```python
from build123d import *

# Parameters (mm, degrees)
SKETCH068_R     = 1.25
PAD036_DEPTH    = 4
PAD037_DEPTH    = 8
POCKET027_DEPTH = 8
PAD038_DEPTH    = 4
PAD039_DEPTH    = 4
PAD040_DEPTH    = 4
PAD041_DEPTH    = 4
SKETCH076_R     = 1.75
POCKET028_DEPTH = 4
FILLET006_R     = 1
CHAMFER_SIZE    = 1


with BuildPart() as part:
    # Sketch068 → Pad036 (new body)
    with BuildSketch(Plane.XY):
        Polygon((0, 0), (-44, 0), (-44, -5), (-32, -5), (-32, -28), (-44, -28), (-44, -33), (0, -33), (0, -28), (-12, -28), (-12, -5), (0, -5), align=None)
        with Locations((-6, -1.8)):
            Circle(SKETCH068_R, mode=Mode.SUBTRACT)
        with Locations((-38, -31.2)):
            Circle(SKETCH068_R, mode=Mode.SUBTRACT)
        with Locations((-6, -31.2)):
            Circle(SKETCH068_R, mode=Mode.SUBTRACT)
        with Locations((-38, -1.8)):
            Circle(SKETCH068_R, mode=Mode.SUBTRACT)
    extrude(amount=PAD036_DEPTH)

    # Sketch069 → Pad037 (join)
    with BuildSketch(Plane.XY.offset(4)):
        Polygon((0, 0), (-44, 0), (-44, -5), (-31, -5), (-31, -28), (-44, -28), (-44, -33), (0, -33), (0, -28), (-13, -28), (-13, -5), (0, -5), align=None)
    extrude(amount=PAD037_DEPTH)

    # Sketch070 → Pocket027 (cut)
    with BuildSketch(Plane.XY.offset(3)):
        Polygon((-42.5, -1.5), (-42.5, -3.5), (-29, -3.5), (-29, -5), (-29, -29.5), (-42.5, -29.5), (-42.5, -31.5), (-1.5, -31.5), (-1.5, -29.5), (-15, -29.5), (-15, -3.5), (-1.5, -3.5), (-1.5, -1.5), align=None)
    extrude(amount=POCKET027_DEPTH, mode=Mode.SUBTRACT)

    # Sketch072 → Pad038 (join)
    with BuildSketch(Plane(origin=(-38, 0, 12), x_dir=(1, 0, 0), z_dir=(0, 0, 1))):
        Polygon((-1.8, 0), (-1.8, 2), (-0.7, 2), (-0.7, 3.5), (-3.8, 3.5), (-3.8, 0), align=None)
        Polygon((0.7, 2), (1.8, 2), (1.8, 0), (3.8, 0), (3.8, 3.5), (0.7, 3.5), align=None)
    extrude(amount=-PAD038_DEPTH)

    # Sketch073 → Pad039 (join)
    with BuildSketch(Plane(origin=(-38, 0, 0), x_dir=(1, 0, 0), z_dir=(0, 0, 1))):
        Polygon((-1.8, 0), (-1.8, 2), (-0.7, 2), (-0.7, 3.5), (-3.8, 3.5), (-3.8, 0), align=None)
        Polygon((0.7, 2), (1.8, 2), (1.8, 0), (3.8, 0), (3.8, 3.5), (0.7, 3.5), align=None)
    extrude(amount=PAD039_DEPTH)

    # Sketch074 → Pad040 (join)
    with BuildSketch(Plane(origin=(-6, 0, 0), x_dir=(1, 0, 0), z_dir=(0, 0, 1))):
        Polygon((-1.8, 0), (-1.8, 2), (-0.7, 2), (-0.7, 3.5), (-3.8, 3.5), (-3.8, 0), align=None)
        Polygon((0.7, 2), (1.8, 2), (1.8, 0), (3.8, 0), (3.8, 3.5), (0.7, 3.5), align=None)
    extrude(amount=PAD040_DEPTH)

    # Sketch075 → Pad041 (join)
    with BuildSketch(Plane(origin=(-6, 0, 12), x_dir=(1, 0, 0), z_dir=(0, 0, 1))):
        Polygon((-1.8, 0), (-1.8, 2), (-0.7, 2), (-0.7, 3.5), (-3.8, 3.5), (-3.8, 0), align=None)
        Polygon((0.7, 2), (1.8, 2), (1.8, 0), (3.8, 0), (3.8, 3.5), (0.7, 3.5), align=None)
    extrude(amount=-PAD041_DEPTH)

    # Sketch076 → Pocket028 (cut)
    with BuildSketch(Plane.YZ):
        with Locations((-30.5, 9.5)):
            Circle(SKETCH076_R)
        with Locations((-30.5, 2.5)):
            Circle(SKETCH076_R)
        with Locations((-2.5, 2.5)):
            Circle(SKETCH076_R)
        with Locations((-2.5, 9.5)):
            Circle(SKETCH076_R)
    extrude(amount=-POCKET028_DEPTH, mode=Mode.SUBTRACT)

    # Fillet006
    fillet006_edges = [part.edges().sort_by_distance(p)[0] for p in [
        (-9.8, 3.5, 2),
        (-2.2, 3.5, 2),
        (-2.2, 3.5, 10),
        (-9.8, 3.5, 10),
        (-34.2, 3.5, 10),
        (-41.8, 3.5, 10),
        (-41.8, 3.5, 2),
        (-34.2, 3.5, 2),
    ]]
    fillet(fillet006_edges, radius=FILLET006_R)

    # Chamfer
    chamfer_edges = [part.edges().sort_by_distance(p)[0] for p in [
        (-5.3, 3.5, 2),
        (-6.7, 3.5, 2),
        (-5.3, 3.5, 10),
        (-6.7, 3.5, 10),
        (-37.3, 3.5, 2),
        (-38.7, 3.5, 2),
        (-38.7, 3.5, 10),
        (-37.3, 3.5, 10),
    ]]
    chamfer(chamfer_edges, length=CHAMFER_SIZE)


with BuildPart() as part_1:
    # Body011 placement: moved
    add(part.part.moved(Location((5, 11, 16.4))))


solid = part_1.part
```
Geometry check sheet. Reference: the model listing, model coordinates, mm. A direction names the side the tool comes from. Round coordinates to 2 decimals unless told otherwise and drop trailing zeros. Order: outer loops, then holes, each group sorted by start corner. A loop starts at its lowest first (then second) coordinate and runs counter-clockwise, first axis right, second up. Notation, with made-up numbers: (-33, 32.25) -> (-3, 32.25) arc R33 cw to (-3, 63.25) -> close; hole circle Ø1 at (36.5, -3). An arc over 180 degrees is marked (long way). Return JSON: item names as keys, results as strings. Group by question number.
Q1. Section check A-A, the plane x = -33. Record the boundary of the cut face in (y, z).
Q2. Release check for a two-part mould opening along X. For faces 5 (the flat face through (-39, -19, 22)), 6 (the flat face through (-30, 13, 24.4)), 7 (the flat face through (-34, 13, 26)) record: released by +X, released by -X, zero draft, split by the parting line, or undercut.
Q3. Gauge pin test, flat ends, axial feed: pin 1 (1.5 mm diameter, centred on x = -26, z = 22.5, fed in from +Y); pin 2 (1.5 mm diameter, centred on y = -1.5, z = 24, fed in from -X); pin 3 (1.5 mm diameter, centred on y = 0.5, z = 21, fed in from +X); pin 4 (2 mm diameter, centred on y = 11.5, z = 26, fed in from +X). Record the tip position at first contact, or that the pin passes through.
Q4. Tool access check on faces 1 (the flat face through (-19, -5, 19.4)), 2 (the cylindrical face through (-0.328, 10.254, 18.372)), 3 (the flat face through (0.2, 14, 18.4)), 4 (the flat face through (-26.5, -5.3, 20.4)). Record the directions out of +Z, -Z, +X, -X, +Y, -Y that give a thin tool (end or side, any length) a straight path to the whole face; none if there is none.
Q5. Section check B-B, the plane y = -2.5. Record the boundary of the cut face in (x, z).
Q6. Section check C-C, the plane x = -17. Record the boundary of the cut face in (y, z).
Q7. Material ranges on probe 1 along Y at (x, z) = (-1, 17.3); probe 2 along X at (y, z) = (9.2, 19); probe 3 along Y at (x, z) = (-1, 19.5), recorded low to high. Write a range as from..to.
Q8. Section check D-D, the plane z = 22.25. Record the boundary of the cut face in (x, y), plus the area to 3 significant figures.
Numbers:
{
 "1": {"outline": "(-22, 16.4) -> (-21.45, 16.4) -> (-21.45, 20.4) -> (-20.5, 20.4) -> (-20.5, 27.4) -> (-18.5, 27.4) -> (-18.5, 19.4) -> (-18.95, 19.4) -> (-18.95, 16.4) -> (-17, 16.4) -> (-17, 28.4) -> (-22, 28.4) -> close; (6, 16.4) -> (7.95, 16.4) -> (7.95, 19.4) -> (7.5, 19.4) -> (7.5, 27.4) -> (9.5, 27.4) -> (9.5, 20.4) -> (10.45, 20.4) -> (10.45, 16.4) -> (11, 16.4) -> (11, 28.4) -> (6, 28.4) -> close"},
 "2": {"face 5": "released by -X", "face 6": "zero draft", "face 7": "undercut"},
 "3": {"pin 1": "y = 11", "pin 2": "x = -26", "pin 3": "x = -7", "pin 4": "x = 5"},
 "4": {"face 1": "none", "face 2": "-Z", "face 3": "+Z, -Z, +Y", "face 4": "+Z, -X"},
 "5": {"outline": "(-27, 16.4) -> (-7, 16.4) -> (-7, 20.4) -> (-8, 20.4) -> (-8, 28.4) -> (-26, 28.4) -> (-26, 20.4) -> (-27, 20.4) -> close; hole (-24, 19.4) -> (-10, 19.4) -> (-10, 27.4) -> (-24, 27.4) -> close"},
 "6": {"outline": "(-22, 16.4) -> (11, 16.4) -> (11, 28.4) -> (-22, 28.4) -> close; hole (-20.5, 19.4) -> (9.5, 19.4) -> (9.5, 27.4) -> (-20.5, 27.4) -> close"},
 "7": {"probe 1": "-22..-21.45, -18.95..-17, 6..7.95, 10.45..11", "probe 2": "-39..-34.25, -31.75..-2.25, 0.25..1", "probe 3": "-22..-21.45, -18.5..-17, 6..7.5, 10.45..11"},
 "8": {"outline": "(-39, -22) -> (5, -22) -> (5, -17) -> (-8, -17) -> (-8, 6) -> (5, 6) -> (5, 11) -> (-39, 11) -> (-39, 6) -> (-26, 6) -> (-26, -17) -> (-39, -17) -> close; hole (-37.5, -20.5) -> (3.5, -20.5) -> (3.5, -18.5) -> (-10, -18.5) -> (-10, 7.5) -> (3.5, 7.5) -> (3.5, 9.5) -> (-37.5, 9.5) -> (-37.5, 7.5) -> (-24, 7.5) -> (-24, -18.5) -> (-37.5, -18.5) -> close", "area": "326 mm^2"}
}
